from build123d import *

# Parameters (mm, degrees)
SKETCH1_W      = 76.2
SKETCH1_H      = 152.4
EXTRUDE1_DEPTH = 25.4
SKETCH2_W      = 25.4
SKETCH2_H      = 25.4
EXTRUDE2_DEPTH = 5
SKETCH3_W      = 8.382
SKETCH3_H      = 25.4
EXTRUDE3_DEPTH = 25
SKETCH4_W      = 25.4
SKETCH4_H      = 25.4
EXTRUDE4_DEPTH = 5
SKETCH5_W      = 8.382
SKETCH5_H      = 25.4
EXTRUDE5_DEPTH = 25


with BuildPart() as part:
    # Sketch1 → Extrude1 (new body)
    with BuildSketch(Plane(origin=(0, 0, 0), x_dir=(1, 0, 0), z_dir=(0, 1, 0))):
        Rectangle(SKETCH1_W, SKETCH1_H)
    extrude(amount=EXTRUDE1_DEPTH)

    # Sketch2 → Extrude2 (add)
    with BuildSketch(Plane.ZY.offset(38.1)):
        with Locations((-63.5, 12.7)):
            Rectangle(SKETCH2_W, SKETCH2_H)
    extrude(amount=EXTRUDE2_DEPTH)

    # Sketch3 → Extrude3 (add)
    with BuildSketch(Plane.ZY.offset(43.1)):
        with Locations((-63.627, 12.7)):
            Rectangle(SKETCH3_W, SKETCH3_H)
    extrude(amount=EXTRUDE3_DEPTH)

    # Sketch4 → Extrude4 (add)
    with BuildSketch(Plane.ZY.offset(38.1)):
        with Locations((-12.7, 12.7)):
            Rectangle(SKETCH4_W, SKETCH4_H)
    extrude(amount=EXTRUDE4_DEPTH)

    # Sketch5 → Extrude5 (add)
    with BuildSketch(Plane.ZY.offset(43.1)):
        with Locations((-12.827, 12.7)):
            Rectangle(SKETCH5_W, SKETCH5_H)
    extrude(amount=EXTRUDE5_DEPTH)


solid = part.part
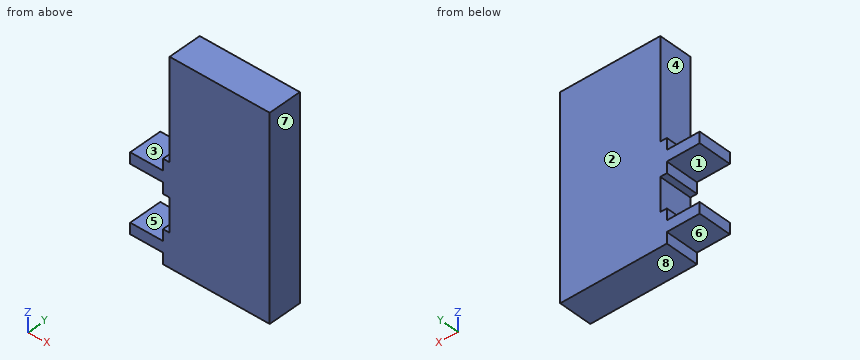
Geometry: final body of the model. Coordinates: model frame, mm. Face numbers are marked on the shaded views. A direction names the side the tool comes from. Round coordinates to 2 decimals unless told otherwise and drop trailing zeros. Loops run counter-clockwise (first coordinate to the right, second up) from the corner with the lowest first, then second, coordinate; pieces in that order, holes last. Notation, with made-up numbers: M 77,70 L 104,70 A17 ccw 104,93 Z; hole C 72,32.5 d6. An arc over 180 degrees is marked long. One line per question, with ' | ' between items.
(1) Cut plane B-B on y = 8.75. Return the cut outline in (x, z), plus the area to 3 significant figures.
Check result:
outline: M -68.1,-67.82 L -43.1,-67.82 L -43.1,-76.2 L 38.1,-76.2 L 38.1,76.2 L -38.1,76.2 L -38.1,0 L -43.1,0 L -43.1,-8.64 L -68.1,-8.64 L -68.1,-17.02 L -43.1,-17.02 L -43.1,-25.4 L -38.1,-25.4 L -38.1,-50.8 L -43.1,-50.8 L -43.1,-59.44 L -68.1,-59.44 Z | area: 12,300 mm2
(2) Cut plane A-A on x = -54. Return the cut outline in (y, z).
Check result:
outline: M 0,-67.82 L 25.4,-67.82 L 25.4,-59.44 L 0,-59.44 Z; M 0,-17.02 L 25.4,-17.02 L 25.4,-8.64 L 0,-8.64 Z
(3) Cut plane D-D on z = 29. Return the cut outline in (x, y), plus the area to 3 significant figures.
Check result:
outline: M -38.1,0 L 38.1,0 L 38.1,25.4 L -38.1,25.4 Z | area: 1,940 mm2
(4) Contact query for flat-ended pins moving along their axis: P1, Ø4, axis at x = -40.5, y = 15, coming from the +Z side; P2, Ø1.5, axis at y = 14, z = 58.5, coming from the -X side; P3, Ø2.5, axis at y = 10, z = -4, coming from the -X side. Output: stop coordinate, or through.
Check result:
P1: stops at z = 0 | P2: stops at x = -38.1 | P3: stops at x = -43.1
(5) Pull-direction query (Z, two-part tool) for the marked faces 1, 2 and 3; classes: +Z half, -Z half, draft (parallel to the pull), parting line (faces both ways), or undercut.
Check result:
face 1: undercut | face 2: draft | face 3: +Z half
(6) Material intervals for line 1 along Z through (x, y) = (-56.5, 4.25); line 2 along Z through (x, y) = (-40, 16.5); line 3 along X through (y, z) = (20.5, -27), sorted ascending. Write a range as from..to.
Check result:
line 1: z = -67.82..-59.44, -17.02..-8.64 | line 2: z = -76.2..-50.8, -25.4..0 | line 3: x = -38.1..38.1
(7) Cut plane C-C on z = -52.5. Return the cut outline in (x, y), plus the area to 3 significant figures.
Check result:
outline: M -43.1,0 L 38.1,0 L 38.1,25.4 L -43.1,25.4 Z | area: 2,060 mm2
(8) Access query for the marked faces 4, 5, 6, 7 and 8. Directions: +Z, -Z, +X, -X, +Y, -Y. A direction counts if a zero-diameter tool reaches every point of the face in a straight line with its end or side. Return the directions, or none.
Check result:
face 4: +Z, -X, +Y, -Y | face 5: -X, +Y, -Y | face 6: -Z, -X, +Y, -Y | face 7: +Z, -Z, +X, +Y, -Y | face 8: -Z, +X, -X, +Y, -Y
